from build123d import *

# Parameters (mm, degrees)
BOSS_EXTRUDE1_DEPTH = 10


with BuildPart() as part:
    # Sketch1 → Boss-Extrude1 (new body)
    with BuildSketch(Plane.XY):
        with BuildLine():
            Line((0, 0), (45, 0))
            ThreePointArc((45, 0), (48.535533906, 1.464466094), (50, 5))
            Line((50, 5), (50, 30))
            Line((50, 30), (5, 30))
            ThreePointArc((5, 30), (1.464466094, 28.535533906), (0, 25))
            Line((0, 25), (0, 0))
        make_face()
        with BuildLine():
            Line((15, 19), (35, 19))
            ThreePointArc((35, 19), (39, 15), (35, 11))
            Line((35, 11), (15, 11))
            ThreePointArc((15, 11), (11, 15), (15, 19))
        make_face(mode=Mode.SUBTRACT)
    extrude(amount=BOSS_EXTRUDE1_DEPTH)


solid = part.part
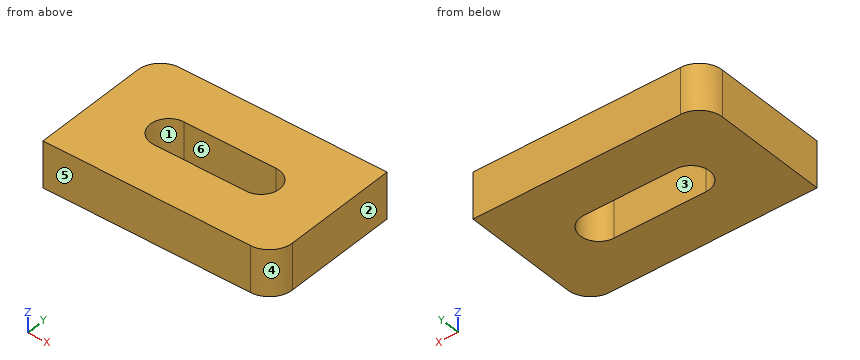
Design review of the part built by this model. Coordinates are the model's own, in mm. Face numbers are marked on the shaded views. A direction names the side the tool comes from. Give positions to 0.01 mm unless a question says otherwise; leave off trailing zeros. Write each loop counter-clockwise with the first axis right and the second up, starting at its lowest first coordinate (ties: lowest second). Pieces come first, ordered by that corner, then holes. Notation, with made-up numbers: M 14.5,63.5 L 48.5,63.5 A8 ccw 48.5,74.5 Z; hole C -30,-11.75 d11. An arc over 180 degrees is marked long. Return JSON: item names as keys, results as strings. Group by question number.
Item 1: Wall thickness on line 1 along Y through (x, z) = (34.5, 2.5); line 2 along X through (y, z) = (14.75, 2.25); line 3 along X through (y, z) = (25.25, 5.75): over which ranges is each line inside the solid? List them lowest first.
Item 2: Take a section at B-B (x = 23.5). Give the boundary of the cut face in (y, z), plus the area to 3 significant figures.
Item 3: Tool access review of the marked faces 5 and 6: name each direction out of +Z, -Z, +X, -X, +Y, -Y from which nothing blocks a thin tool from reaching the whole face with its end or side.
Item 4: Take a section at A-A (y = 15). Give the boundary of the cut face in (x, z).
Item 5: The part is to be moulded in two halves that separate along Y. For the marked faces 1, 2, 3 and 4, say which applies: pulls with the +Y half, pulls with the -Y half, needs draft (parallel to the pull), parting line crosses it, or undercut.
Item 6: Take a section at C-C (z = 6.75). Give the boundary of the cut face in (x, y).
Return value:
{
 "1": {"line 1": "y = 0 to 11, 19 to 30", "line 2": "x = 0 to 11.01, 38.99 to 50", "line 3": "x = 0.01 to 50"},
 "2": {"outline": "M 0,0 L 11,0 L 11,10 L 0,10 Z; M 19,0 L 30,0 L 30,10 L 19,10 Z", "area": "220 mm2"},
 "3": {"face 5": "+Z, -Z, +X, -X, -Y", "face 6": "+Z, -Z"},
 "4": {"outline": "M 0,0 L 11,0 L 11,10 L 0,10 Z; M 39,0 L 50,0 L 50,10 L 39,10 Z"},
 "5": {"face 1": "undercut", "face 2": "needs draft", "face 3": "undercut", "face 4": "pulls with the -Y half"},
 "6": {"outline": "M 0,0 L 45,0 A5 ccw 50,5 L 50,30 L 5,30 A5 ccw 0,25 Z; hole M 15,11 L 35,11 A4 ccw 35,19 L 15,19 A4 ccw Z"}
}
